```python
from build123d import *

# Parameters (mm, degrees)
SKETCH3_R           = 28.5496
BOSS_EXTRUDE1_DEPTH = 56.5404
SKETCH4_R           = 28.5496
BOSS_EXTRUDE2_DEPTH = 28.2702


with BuildPart() as part:
    # Sketch1 → Revolve1 (revolve)
    with BuildSketch(Plane.XY):
        Polygon((-57.785, -28.5496), (-28.2702, -28.5496), (-28.2702, -24.0538), (-57.785, -24.2824), align=None)
        Polygon((57.785, -24.2824), (28.2702, -24.0538), (28.2702, -28.5496), (57.785, -28.5496), align=None)
    revolve(axis=Axis((-57.785, 0, 0), (1, 0, 0)))



with BuildPart() as body_2:
    # Sketch2 → Revolve2 (revolve)
    with BuildSketch(Plane.XY):
        Polygon((24.2824, 57.785), (24.0538, 28.2702), (28.5496, 28.2702), (28.5496, 57.785), align=None)
    revolve(axis=Axis((0, 0, 0), (0, 1, 0)))


with BuildPart() as part_1:
    add(part.part)

    add(body_2.part)  # Boss-Extrude1 merges body 2
    # Sketch3 → Boss-Extrude1 (add)
    with BuildSketch(Plane(origin=(-28.2702, 0, 0), x_dir=(0, 0, -1), z_dir=(1, 0, 0))):
        Circle(SKETCH3_R)
    extrude(amount=BOSS_EXTRUDE1_DEPTH)

    # Sketch4 → Boss-Extrude2 (add)
    with BuildSketch(Plane.XZ.offset(-28.2702)):
        Circle(SKETCH4_R)
    extrude(amount=BOSS_EXTRUDE2_DEPTH)

    # Sketch5 → Cut-Revolve1 (revolve, cut)
    with BuildSketch(Plane.XY):
        Polygon((-57.785, -24.2824), (-28.2702, -24.0538), (-28.2702, -20.447), (28.2702, -20.447), (28.2702, -24.0538), (57.785, -24.2824), (57.785, 0), (-57.785, 0), align=None)
    revolve(axis=Axis((57.785, 0, 0), (-1, 0, 0)), mode=Mode.SUBTRACT)

    # Sketch6 → Cut-Revolve2 (revolve, cut)
    with BuildSketch(Plane.XY):
        Polygon((24.2824, 57.785), (24.0538, 28.2702), (20.447, 28.2702), (20.447, 0), (0, 0), (0, 57.785), align=None)
    revolve(axis=Axis((0, 0, 0), (0, 1, 0)), mode=Mode.SUBTRACT)


solid = part_1.part
```
Work out the finished part from the listing and answer in its coordinate system (mm). A direction names the side the tool comes from. Give positions to 0.01 mm unless a question says otherwise; leave off trailing zeros. Loops run counter-clockwise (first coordinate to the right, second up) from the corner with the lowest first, then second, coordinate; pieces in that order, holes last. Notation, with made-up numbers: (-40, -19.5) -> (9, -19.5) arc R16 ccw to (9, -6.5) -> close; hole circle Ø4 at (57, -34.75). An arc over 180 degrees is marked (long way). Put each result on its own line as item: value. Start each with the question number.
Item 1: Find the intervals of material crossed by L1, parallel to Z at x = 30, y = -1; L2, parallel to Z at x = 0, y = 19; L3, parallel to Y at x = -11.5, z = 0, in increasing order. Write a range as [from, to].
Item 2: Which of the six approach directions +Z, -Z, +X, -X, +Y, -Y give full straight-line access (tool end or side, diameter ignored) to faces 1 (the face through (8.3, 57.785, -23.4)), 2 (the face through (9.435, 20.219, 18.14))?
Item 3: The mould has two halves that part along Z. Classify faces 3 (the face through (-28.52, 35.72, 1.26)), 4 (the face through (-57.785, 8.3, -23.4)), 5 (the face through (0.396, -19.503, 6.142)): released by +Z, released by -Z, zero draft, split by the parting line, or undercut.
Item 4: The part is cut by section A-A (z = 9.5). State how many separate pieces and enclosed holes the cut face has, then the cut area to 3 significant figures.
Item 5: The part is cut by section C-C (y = 40.5). Give the vertices of the cut face in (x, z), then the cut area to 3 significant figures.
Item 6: Each of these flat-tipped pins is pushed along its axis until it touches: P1, Ø3, axis at x = 39, z = -21.5, coming from the +Y side; P2, Ø12, axis at x = -16, y = 11.5, coming from the +Z side; P3, Ø24, axis at y = 6, z = 4, coming from the +X side; P4, Ø1.2, axis at y = 22, z = 1, coming from the +X side. Where does it stop, or does it pass through?
Item 7: The part is cut by section B-B (x = 37). Give the vertices of the cut face in (y, z).
Answers below:
1. L1: [-28.53, -24.05], [24.05, 28.53]
1. L2: [-28.55, -20.45], [20.45, 28.55]
1. L3: [-28.55, -20.45]
2. face 1: +Z, -Z, +X, -X, +Y
2. face 2: +Y
3. face 3: split by the parting line
3. face 4: zero draft
3. face 5: undercut
4. separate pieces: 3
4. enclosed holes: 0
4. area: 1,530 mm2
5. outline: circle Ø57.1 at (0, 0); hole circle Ø48.3 at (0, 0)
5. area: 729 mm2
6. P1: y = 20.37
6. P2: z = 28.01
6. P3: through
6. P4: x = 28.27
7. outline: circle Ø57.1 at (0, 0); hole circle Ø48.24 at (0, 0)
